from build123d import *

# Parameters (mm, degrees)
BOSS_EXTRUDE1_DEPTH      = 5
M3_CLEARANCE_HOLE1_D     = 3.4
M3_CLEARANCE_HOLE1_DEPTH = 5
M3_CLEARANCE_HOLE1_TIP   = 1.021463052
SKETCH4_R                = 3.975
BOSS_EXTRUDE2_DEPTH      = 36.5
SKETCH5_R                = 3.025
CUT_EXTRUDE1_DEPTH       = 2


with BuildPart() as part:
    # Sketch1 → Boss-Extrude1 (new body)
    with BuildSketch(Plane(origin=(0, 0, 0), x_dir=(1, 0, 0), z_dir=(0, 1, 0))):
        with BuildLine():
            Line((-9, 5), (9, 5))
            ThreePointArc((9, 5), (14, 0), (9, -5))
            Line((9, -5), (-9, -5))
            ThreePointArc((-9, -5), (-14, 0), (-9, 5))
        make_face()
    extrude(amount=BOSS_EXTRUDE1_DEPTH)

    # M3 Clearance Hole1
    with Locations(Plane(origin=(0, 5, 0), x_dir=(1, 0, 0), z_dir=(0, 1, 0))):
        with Locations((-9.5, 0), (9.5, 0)):
            Hole(M3_CLEARANCE_HOLE1_D / 2, depth=M3_CLEARANCE_HOLE1_DEPTH)
            with Locations((0, 0, -(M3_CLEARANCE_HOLE1_DEPTH + M3_CLEARANCE_HOLE1_TIP / 2))):  # 118° drill point
                Cone(0, M3_CLEARANCE_HOLE1_D / 2, M3_CLEARANCE_HOLE1_TIP, mode=Mode.SUBTRACT)

    # Sketch4 → Boss-Extrude2 (add)
    with BuildSketch(Plane(origin=(0, 5, 0), x_dir=(1, 0, 0), z_dir=(0, 1, 0))):
        Circle(SKETCH4_R)
    extrude(amount=BOSS_EXTRUDE2_DEPTH)

    # Sketch5 → Cut-Extrude1 (cut)
    with BuildSketch(Plane(origin=(0, 41.5, 0), x_dir=(1, 0, 0), z_dir=(0, 1, 0))):
        Circle(SKETCH5_R)
    extrude(amount=-CUT_EXTRUDE1_DEPTH, mode=Mode.SUBTRACT)


solid = part.part
Model file for the job. Use its own axes, mm. A direction names the side the tool comes from. Round coordinates to 2 decimals unless told otherwise and drop trailing zeros. Loops run counter-clockwise (first coordinate to the right, second up) from the corner with the lowest first, then second, coordinate; pieces in that order, holes last.
1. Band-saw the part on B-B, the plane x = 0. List the corners of the cut face in (y, z) (3 decimals), and give its area (3 significant figures).
Check values:
outline: (0, -5) - (5, -5) - (5, -3.975) - (41.5, -3.975) - (41.5, -3.025) - (39.5, -3.025) - (39.5, 3.025) - (41.5, 3.025) - (41.5, 3.975) - (5, 3.975) - (5, 5) - (0, 5) - close
area: 328 mm2
2. Mould opens along Z. For faces 3 (the cylindrical face through (-0.86, 22.99, 3.88)), 4 (the flat face through (0, 41.5, 3.2)), 5 (the flat face through (0, 39.5, 0)), 6 (the cylindrical face through (9.87, 2.46, 1.66)) say: +Z half, -Z half, draft (parallel to the pull), parting line (faces both ways), or undercut.
Check values:
face 3: parting line
face 4: draft
face 5: undercut
face 6: undercut
3. Band-saw the part on A-A, the plane z = 0. List the corners of the cut face in (x, y) (3 decimals).
Check values:
outline: (-14, 0) - (-11.2, 0) - (-11.2, 5) - (-14, 5) - close; (-7.8, 0) - (7.8, 0) - (7.8, 5) - (3.975, 5) - (3.975, 41.5) - (3.025, 41.5) - (3.025, 39.5) - (-3.025, 39.5) - (-3.025, 41.5) - (-3.975, 41.5) - (-3.975, 5) - (-7.8, 5) - close; (11.2, 0) - (14, 0) - (14, 5) - (11.2, 5) - close
4. Band-saw the part on C-C, the plane x = 9.5. List the corners of the cut face in (y, z), and give its area (3 significant figures).
Check values:
outline: (0, -4.97) - (5, -4.97) - (5, -1.7) - (0, -1.7) - close; (0, 1.7) - (5, 1.7) - (5, 4.97) - (0, 4.97) - close
area: 32.7 mm2
5. Band-saw the part on D-D, the plane y = 38. List the corners of the cut face in (x, z) (3 decimals), and give its area (3 significant figures).
Check values:
outline: circle Ø7.95 at (0, 0)
area: 49.6 mm2
6. Wall check: probe 1 along X at (y, z) = (40.6, 0) (3 decimals); probe 2 along X at (y, z) = (31.5, 0) (3 decimals). Give the ranges that are in metal, low to high.
Check values:
probe 1: x = -3.975 to -3.025, 3.025 to 3.975
probe 2: x = -3.975 to 3.975
7. Drop flat-ended pins along their axis: P1, Ø2, axis at x = 11, z = 2, coming from the +Y side; P2, Ø5, axis at x = 0, z = 0, coming from the +Y side; P3, Ø6, axis at y = 30, z = 1, coming from the +X side (3 decimals). Give the stop position or say it passes through.
Check values:
P1: stops at y = 5
P2: stops at y = 39.5
P3: stops at x = 3.975
8. Tool access for faces 1 (the cylindrical face through (2.794, 40.514, 1.159)), 2 (the flat face through (0, 0, 0)): list every direction of +Z, -Z, +X, -X, +Y, -Y with a clear straight run to the whole face (end or side of a thin tool).
Check values:
face 1: +Y
face 2: +Z, -Z, +X, -X, -Y
